Autodesk Inventor part; units mm, degrees
ref_plane "YZ Plane" through (0, 0, 0) normal (1, 0, 0) x (0, 1, 0)
ref_plane "XZ Plane" through (0, 0, 0) normal (0, 1, 0) x (-1, 0, 0)
ref_plane "XY Plane" through (0, 0, 0) normal (0, 0, 1) x (1, 0, 0)
sketch "Sketch1" plane through (0, 0, 0) normal (0, 1, 0) x (-1, 0, 0)
  line L0 (-32.25, -38.75) -> (32.25, -38.75)
  line L1 (32.25, -38.75) -> (32.25, 38.75)
  line L2 (32.25, 38.75) -> (-32.25, 38.75)
  line L3 (-32.25, 38.75) -> (-32.25, -38.75)
  line L4 (-32.25, -38.75) -> (32.25, 38.75) construction
  line L5 (32.25, -38.75) -> (-32.25, 38.75) construction
  point P0 (0, 0)
  dimension "d0" = 64.5
  dimension "d1" = 77.5
extrude "Extrusion1" add sketch "Sketch1" along normal blind 3
sketch "Sketch4" plane through (-32.25, 0, -38.75) normal (-1, 0, 0) x (0, 0, 1)
  line L0 (0, 3) -> (77.5, 3)
  line L1 (0, 0) -> (77.5, 0)
  line L2 (31, 3) -> (46, 3)
  line L3 (46, 3) -> (46, 0)
  line L4 (46, 0) -> (31, 0)
  line L5 (31, 0) -> (31, 3)
  line L6 (0, 0) -> (0, 3)
  line L7 (77.5, 0) -> (77.5, 3)
  point P0 (38.75, 0)
  dimension "d17" = 15
  dimension "d18" = 31
  dimension "d19" = 31.5
extrude "Extrusion3" add sketch "Sketch4" along normal blind 15 contours L0 L3 L1 L5
sketch "Sketch5" plane through (0, 3, 0) normal (0, 1, 0) x (1, 0, 0)
  circle A0 centre (-39.25, 0.25) radius 5
  line L0 (-32.25, -7.25) -> (-47.25, -7.25)
  line L1 (-32.25, 7.75) -> (-47.25, 7.75)
  line L2 (-47.25, -7.25) -> (-47.25, 7.75)
  point P0 (0, 0)
  dimension "d22" = 10
  dimension "d34" = 7.5
  dimension "d35" = 7.5
  dimension "d36" = 8
extrude "Extrusion4" cut sketch "Sketch5" against normal up to surface (3 mm away)
fillet "Fillet1" radius 6 2 edges at (-47.25, 1.5, 7.25) (-47.25, 1.5, -7.75)
sketch "Sketch6" plane through (0, 0, 0) normal (0, -1, 0) x (1, 0, 0)
  line L0 (-19.1342, -27.716) -> (23.9028, -27.716)
  line L1 (24.9028, -26.716) -> (24.9028, -26.3695)
  line L2 (23.9028, -25.3695) -> (-19.1342, -25.3695)
  line L3 (-20.1342, -26.3695) -> (-20.1342, -26.716)
  arc A0 (-20.1342, -26.716) -> (-19.1342, -27.716) centre (-19.1342, -26.716) ccw
  arc A1 (-19.1342, -25.3695) -> (-20.1342, -26.3695) centre (-19.1342, -26.3695) ccw
  arc A2 (23.9028, -27.716) -> (24.9028, -26.716) centre (23.9028, -26.716) ccw
  arc A3 (24.9028, -26.3695) -> (23.9028, -25.3695) centre (23.9028, -26.3695) ccw
  line L4 (-19.1342, -1.2568) -> (23.9028, -1.2568)
  line L5 (24.9028, -0.2568) -> (24.9028, 0.0896)
  line L6 (23.9028, 1.0896) -> (-19.1342, 1.0896)
  line L7 (-20.1342, 0.0896) -> (-20.1342, -0.2568)
  arc A4 (-20.1342, -0.2568) -> (-19.1342, -1.2568) centre (-19.1342, -0.2568) ccw
  arc A5 (-19.1342, 1.0896) -> (-20.1342, 0.0896) centre (-19.1342, 0.0896) ccw
  arc A6 (23.9028, -1.2568) -> (24.9028, -0.2568) centre (23.9028, -0.2568) ccw
  arc A7 (24.9028, 0.0896) -> (23.9028, 1.0896) centre (23.9028, 0.0896) ccw
  line L8 (-19.1342, 21.9427) -> (23.9028, 21.9427)
  line L9 (24.9028, 22.9427) -> (24.9028, 23.2892)
  line L10 (23.9028, 24.2892) -> (-19.1342, 24.2892)
  line L11 (-20.1342, 23.2892) -> (-20.1342, 22.9427)
  arc A8 (-20.1342, 22.9427) -> (-19.1342, 21.9427) centre (-19.1342, 22.9427) ccw
  arc A9 (-19.1342, 24.2892) -> (-20.1342, 23.2892) centre (-19.1342, 23.2892) ccw
  arc A10 (23.9028, 21.9427) -> (24.9028, 22.9427) centre (23.9028, 22.9427) ccw
  arc A11 (24.9028, 23.2892) -> (23.9028, 24.2892) centre (23.9028, 23.2892) ccw
  point P0 (0, 0)
  dimension "d27" = 1
  dimension "d28" = 1
  dimension "d29" = 1
extrude "Extrusion5" cut sketch "Sketch6" against normal up to surface (3 mm away)
sketch "Sketch7" plane through (0, 3, 0) normal (0, 1, 0) x (1, 0, 0)
  circle A0 centre (-30.232, -37.014) radius 3.5
  line L0 (-32.25, -38.75) -> (32.25, -38.75)
  line L1 (-32.25, -7.25) -> (-32.25, -38.75)
  circle A1 centre (30.232, -37.014) radius 3.5
  circle A2 centre (-30.232, 37.014) radius 3.5
  circle A3 centre (30.232, 37.014) radius 3.5
  line L2 (32.25, 38.75) -> (-32.25, 38.75)
  line L3 (-32.25, 38.75) -> (-32.25, 7.75)
  line L4 (32.25, -38.75) -> (32.25, 38.75)
  point P0 (0, 0)
  dimension "d37" = 7
  dimension "d38" = 1.736
  dimension "d39" = 2.018
  dimension "d40" = 7
  dimension "d41" = 7
  dimension "d42" = 7
  dimension "d43" = 1.736
  dimension "d44" = 2.018
  dimension "d45" = 1.736
  dimension "d46" = 2.018
  dimension "d47" = 1.736
  dimension "d48" = 2.018
extrude "Extrusion6" add sketch "Sketch7" against normal up to surface (3 mm away)
sketch "Sketch8" plane through (0, 3, 0) normal (0, 1, 0) x (1, 0, 0)
  circle A0 centre (30.232, -37.014) radius 1.6
  circle A1 centre (-30.232, -37.014) radius 1.6
  circle A2 centre (-30.232, 37.014) radius 1.6
  circle A3 centre (30.232, 37.014) radius 1.6
  point P0 (0, 0)
  dimension "d51" = 3.2
  dimension "d52" = 3.2
  dimension "d53" = 3.2
  dimension "d54" = 3.2
extrude "Extrusion7" cut sketch "Sketch8" against normal up to surface (3 mm away)
chamfer "Chamfer1" distance 1 angle 45 4 edges at (-31.832, 3, 37.014) (28.632, 3, -37.014) (-31.832, 3, -37.014) (28.632, 3, 37.014)
properties part number "_3DPrint"
Check sheet for the modelled part. Datum: model origin and axes. Units: mm. A direction names the side the tool comes from. Round coordinates to 2 decimals unless told otherwise and drop trailing zeros. Loops run counter-clockwise (first coordinate to the right, second up) from the corner with the lowest first, then second, coordinate; pieces in that order, holes last. Notation, with made-up numbers: (77, -20.5) -> (122, -20.5) arc R15 ccw to (122, -10.5) -> close; hole circle Ø2 at (20, 24.5). An arc over 180 degrees is marked (long way). Write item = value, one per line. Start each with the question number.
1) Set-up check for faces 1 (the flat face through (3, 3, 10)), 2 (the flat face through (3, 1, 24.289)), 3 (the flat face through (0, 1, -38.75)), 4 (the flat face through (-32.25, 1, -21)): record each of +Z, -Z, +X, -X, +Y, -Y from which the full face is reachable in a straight line by a thin tool's end or side.
2) Sectioned sample at B-B, the plane x = -39.25. Record the cut outline in (y, z).
3) Release check for a two-part mould opening along Z. For faces 5 (the flat face through (-32.25, 1, 21)), 6 (the flat face through (0, 1, 38.75)), 7 (the flat face through (3, 0, 10)) record: released by +Z, released by -Z, zero draft, split by the parting line, or undercut.
4) Sectioned sample at C-C, the plane z = 8.5. Record the cut outline in (x, y).
5) Sectioned sample at D-D, the plane y = 0.6. State how many separate pieces and enclosed holes the cut face has, plus the area to 3 significant figures.
6) Thickness scan on probe 1 along Z at (x, y) = (21, 0.65); probe 2 along X at (y, z) = (1.3, -0.25); probe 3 along Z at (x, y) = (-39.25, 1.25). Record the ranges inside material, lowest first.
7) Gauge pin test, flat ends, axial feed: pin 1 Ø1 at (y, z) = (0.5, 21.5) entering from -X; pin 2 Ø0.9 at (x, y) = (6, 1) entering from -Z; pin 3 Ø1.5 at (x, y) = (-38, 1.5) entering from +Z. Record the tip position at first contact, or that the pin passes through.
8) Sectioned sample at A-A, the plane x = -17.5. Record the cut outline in (y, z), plus the area to 3 significant figures.
Results are:
q1.face_1 = +Z, -Z, +X, -X, +Y
q1.face_2 = +Y, -Y
q1.face_3 = -Z, +Y, -Y
q1.face_4 = -X, +Y, -Y
q2.outline = (0, -7.75) -> (3, -7.75) -> (3, -5.25) -> (0, -5.25) -> close; (0, 4.75) -> (3, 4.75) -> (3, 7.25) -> (0, 7.25) -> close
q3.face_5 = undercut
q3.face_6 = released by +Z
q3.face_7 = zero draft
q4.outline = (-32.25, 0) -> (32.25, 0) -> (32.25, 3) -> (-32.25, 3) -> close
q5.separate_pieces = 1
q5.enclosed_holes = 8
q5.area = 4,830 mm^2
q6.probe_1 = -38.75 to -27.72, -25.37 to -1.26, 1.09 to 21.94, 24.29 to 38.75
q6.probe_2 = -47.25 to -44.25, -34.25 to -20.13, 24.9 to 32.25
q6.probe_3 = -7.75 to -5.25, 4.75 to 7.25
q7.pin_1 = -32.25
q7.pin_2 = -38.75
q7.pin_3 = 7.25
q8.outline = (0, -38.75) -> (3, -38.75) -> (3, -27.72) -> (0, -27.72) -> close; (0, -25.37) -> (3, -25.37) -> (3, -1.26) -> (0, -1.26) -> close; (0, 1.09) -> (3, 1.09) -> (3, 21.94) -> (0, 21.94) -> close; (0, 24.29) -> (3, 24.29) -> (3, 38.75) -> (0, 38.75) -> close
q8.area = 211 mm^2
